Geometry: final body of the model. Coordinates: model frame, mm. A direction names the side the tool comes from. Give positions to 0.01 mm unless a question says otherwise; leave off trailing zeros. Write each loop counter-clockwise with the first axis right and the second up, starting at its lowest first coordinate (ties: lowest second). Pieces come first, ordered by that corner, then holes.
```python
from build123d import *

# Parameters (mm, degrees)
SKETCH7_W           = 203.2
SKETCH7_H           = 127
SKETCH7_W_2         = 124.5
SKETCH7_H_2         = 82.199999938
BOSS_EXTRUDE4_DEPTH = 12.7
SKETCH8_W           = 12.7
SKETCH8_H           = 6.35
SKETCH8_W_2         = 6.35
SKETCH8_H_2         = 12.7
BOSS_EXTRUDE5_DEPTH = 12.7
SKETCH10_R          = 9.525
SKETCH10_R_2        = 12.7
SKETCH10_R_3        = 25.4
CUT_EXTRUDE1_DEPTH  = 130.203386179


with BuildPart() as part:
    # Sketch7 → Boss-Extrude4 (new body)
    with BuildSketch(Plane(origin=(0, 0, 0), x_dir=(1, 0, 0), z_dir=(0, 1, 0))):
        Rectangle(SKETCH7_W, SKETCH7_H)
        with Locations((0, 9.700000031)):
            Rectangle(SKETCH7_W_2, SKETCH7_H_2, mode=Mode.SUBTRACT)
    extrude(amount=BOSS_EXTRUDE4_DEPTH)

    # Sketch8 → Boss-Extrude5 (add)
    with BuildSketch(Plane(origin=(0, 0, 0), x_dir=(1, 0, 0), z_dir=(0, 1, 0))):
        Polygon((-101.6, 69.85), (-88.9, 69.85), (-88.9, 63.5), (-101.6, 50.8), (-107.95, 50.8), (-107.95, 63.5), (-107.95, 69.85), align=None)
        with Locations((-57.15, 66.675)):
            Rectangle(SKETCH8_W, SKETCH8_H)
        with Locations((-19.05, 66.675)):
            Rectangle(SKETCH8_W, SKETCH8_H)
        with Locations((19.05, 66.675)):
            Rectangle(SKETCH8_W, SKETCH8_H)
        with Locations((57.15, 66.675)):
            Rectangle(SKETCH8_W, SKETCH8_H)
        with Locations((-104.775, 19.05)):
            Rectangle(SKETCH8_W_2, SKETCH8_H_2)
        with Locations((-104.775, -19.05)):
            Rectangle(SKETCH8_W_2, SKETCH8_H_2)
        Polygon((-101.6, -50.8), (-88.9, -63.5), (-88.9, -69.85), (-101.6, -69.85), (-107.95, -69.85), (-107.95, -63.5), (-107.95, -50.8), align=None)
        Polygon((101.6, 50.8), (88.9, 63.5), (88.9, 69.85), (101.6, 69.85), (107.95, 69.85), (107.95, 63.5), (107.95, 50.8), align=None)
        Polygon((101.6, -69.85), (88.9, -69.85), (88.9, -63.5), (101.6, -50.8), (107.95, -50.8), (107.95, -63.5), (107.95, -69.85), align=None)
        with Locations((104.775, -19.05)):
            Rectangle(SKETCH8_W_2, SKETCH8_H_2)
        with Locations((104.775, 19.05)):
            Rectangle(SKETCH8_W_2, SKETCH8_H_2)
        with Locations((57.15, -66.675)):
            Rectangle(SKETCH8_W, SKETCH8_H)
        with Locations((19.05, -66.675)):
            Rectangle(SKETCH8_W, SKETCH8_H)
        with Locations((-19.05, -66.675)):
            Rectangle(SKETCH8_W, SKETCH8_H)
        with Locations((-57.15, -66.675)):
            Rectangle(SKETCH8_W, SKETCH8_H)
    extrude(amount=BOSS_EXTRUDE5_DEPTH)

    # Sketch10 → Cut-Extrude1 (cut, through all)
    with BuildSketch(Plane(origin=(0, 12.7, 0), x_dir=(1, 0, 0), z_dir=(0, 1, 0))):
        with Locations((0, 50.8)):
            Circle(SKETCH10_R)
        with Locations((-62.25, 9.700000031)):
            Circle(SKETCH10_R_2)
        with Locations((0, -31.399999938)):
            Circle(SKETCH10_R_3)
        with Locations((62.25, 9.700000031)):
            Circle(SKETCH10_R_2)
    extrude(amount=-CUT_EXTRUDE1_DEPTH, mode=Mode.SUBTRACT)


solid = part.part
```
Item 1: Section B-B, the plane z = -42.5. Return the cut outline in (x, y), plus the area to 3 significant figures.
Found:
outline: (-101.6, 0) - (-62.25, 0) - (-62.25, 12.7) - (-101.6, 12.7) - close; (62.25, 0) - (101.6, 0) - (101.6, 12.7) - (62.25, 12.7) - close
area: 999 mm2
Item 2: Section A-A, the plane x = 0. Return the cut outline in (y, z) (3 decimals), plus the area to 3 significant figures.
Found:
outline: (0, -63.5) - (12.7, -63.5) - (12.7, -60.325) - (0, -60.325) - close; (0, 56.8) - (12.7, 56.8) - (12.7, 63.5) - (0, 63.5) - close
area: 125 mm2
Item 3: Reachability of faces 5 (the face through (38, 6, -63.5)), 6 (the face through (-105, 6, 12.7)), 7 (the face through (101.6, 6, -38)), 8 (the face through (74.947, 6.439, -9.421)) from +Z, -Z, +X, -X, +Y, -Y: full face, straight path, thin tool, end or side. Return the list, or none.
Found:
face 5: -Z, +Y, -Y
face 6: -X, +Y, -Y
face 7: +X, +Y, -Y
face 8: +Y, -Y
Item 4: Pin query (flat end, axial travel): pin 1 Ø4 at (y, z) = (11, 3) entering from -X; pin 2 Ø2 at (x, y) = (-41, 8) entering from +Z; pin 3 Ø4 at (x, y) = (33, 9.5) entering from -Z. Return the tip coordinate at first contact, or that it passes through.
Found:
pin 1: stops at x = -101.6
pin 2: stops at z = 63.5
pin 3: stops at z = -63.5
Item 5: Line query: L1, parallel to X at y = 10.5, z = -38; L2, parallel to Z at x = -45.5, y = 6.5; L3, parallel to X at y = 12, z = 18.5. Output: solid intervals per line, ascending.
Found:
L1: x = -101.6 to -62.25, 62.25 to 101.6
L2: z = -63.5 to -50.8, 31.4 to 63.5
L3: x = -107.95 to -62.25, 62.25 to 107.95
Item 6: Pull-direction query (X, two-part tool) for faces 1 (the face through (107.95, 6, 19)), 2 (the face through (19, 6, -69.85)), 3 (the face through (12.7, 6, -67)), 4 (the face through (-107.95, 6, -19)); classes: +X half, -X half, draft (parallel to the pull), parting line (faces both ways), or undercut.
Found:
face 1: +X half
face 2: draft
face 3: undercut
face 4: -X half
